Check sheet for the drawn part. Datum: minimum x, y, z corner. Units: mm. Give positions to 0.01 mm unless a question says otherwise; leave off trailing zeros. Write each loop counter-clockwise with the first axis right and the second up, starting at its lowest first coordinate (ties: lowest second). Pieces come first, ordered by that corner, then holes. Notation, with made-up numbers: (-8, 28) - (3, 28) arc R11 cw to (3, 46) - close; hole circle Ø6 at (75.25, 83). An arc over 180 degrees is marked (long way). Answer as a JSON object with one key per item and string values. Group by question number.
Item 1: Scan lines: line 1 along X through (y, z) = (0.45, 8.5) (1 decimal); line 2 along Z through (x, y) = (16, 0.7) (1 decimal); line 3 along Z through (x, y) = (24, 0.6) (1 decimal). Record each from-to range of solid material in increasing order. Write a range as [from, to].
Item 2: Sectioned sample at A-A, the plane z = 8. Record the boundary of the cut face in (x, y) (1 decimal).
Item 3: Sectioned sample at C-C, the plane x = 9.25. Record the boundary of the cut face in (y, z) (1 decimal).
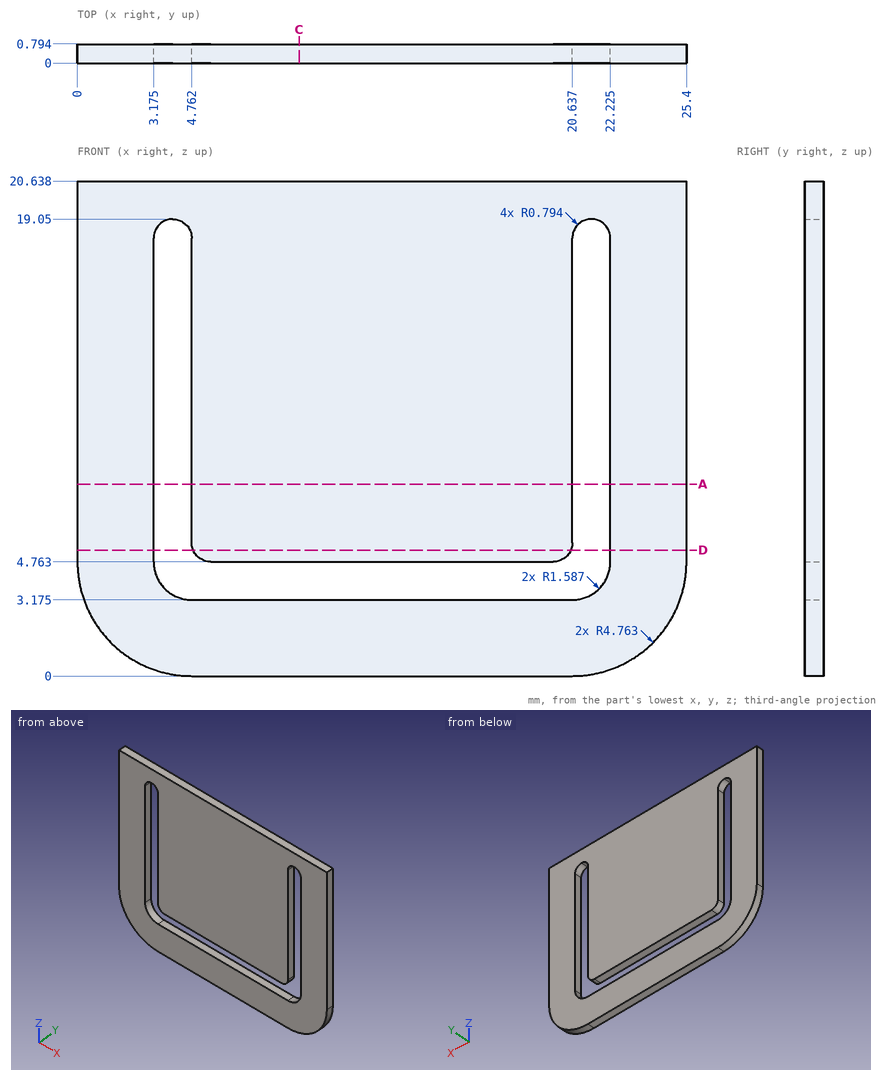
Geometry check:
{
 "1": {"line 1": "[0, 3.2], [4.8, 20.6], [22.2, 25.4]", "line 2": "[0, 3.2], [4.8, 20.6]", "line 3": "[1.4, 20.6]"},
 "2": {"outline": "(0, 0) - (3.2, 0) - (3.2, 0.8) - (0, 0.8) - close; (4.8, 0) - (20.6, 0) - (20.6, 0.8) - (4.8, 0.8) - close; (22.2, 0) - (25.4, 0) - (25.4, 0.8) - (22.2, 0.8) - close"},
 "3": {"outline": "(0, 0) - (0.8, 0) - (0.8, 3.2) - (0, 3.2) - close; (0, 4.8) - (0.8, 4.8) - (0.8, 20.6) - (0, 20.6) - close"}
}
